Part model, mm, in its own coordinate system. A direction names the side the tool comes from. Round coordinates to 2 decimals unless told otherwise and drop trailing zeros. Write each loop counter-clockwise with the first axis right and the second up, starting at its lowest first coordinate (ties: lowest second). Pieces come first, ordered by that corner, then holes.
from build123d import *

# Parameters (mm, degrees)
SKETCH1_W          = 50.8
SKETCH1_H          = 50.8
EXTRUDE1_DEPTH     = 7.9375
SKETCH6_R          = 11.1125
CUT_EXTRUDE2_DEPTH = 8.255
SKETCH3_R          = 6.35
EXTRUDE3_DEPTH     = 6.35
CHAMFER1_SIZE      = 9.525


with BuildPart() as part:
    # Sketch1 → Extrude1 (new body, symmetric)
    with BuildSketch(Plane.XY):
        Rectangle(SKETCH1_W, SKETCH1_H)
    extrude(amount=EXTRUDE1_DEPTH, both=True)

    # Sketch6 → Cut-Extrude2 (cut)
    with BuildSketch(Plane.XY.offset(7.9375)):
        Circle(SKETCH6_R)
    extrude(amount=-CUT_EXTRUDE2_DEPTH, mode=Mode.SUBTRACT)

    # Sketch3 → Extrude3 (add)
    with BuildSketch(Plane.ZY.offset(25.4)):
        with Locations(Location((0, 0, 0), (0, 0, 90))):  # turned: the seam where the file's is
            Circle(SKETCH3_R)
    extrude3 = extrude(amount=EXTRUDE3_DEPTH)

    # Mirror2: Extrude3 across plane
    add(extrude3.mirror(Plane(origin=(0, 0, 0), x_dir=(0, 0, 1), z_dir=(1, 0, 0))))

    # Chamfer1
    chamfer1_edges = [part.edges().sort_by_distance(p)[0] for p in [
        (0, 25.4, -7.9375),
        (0, -25.4, -7.9375),
    ]]
    chamfer(chamfer1_edges, length=CHAMFER1_SIZE)


solid = part.part
Q1. Tool access for faces 4 (the flat face through (0, 0, -0.318)), 5 (the cylindrical face through (28.53, -5.04, 3.86)), 6 (the flat face through (-0.36, -20.57, -3.24)): list every direction of +Z, -Z, +X, -X, +Y, -Y with a clear straight run to the whole face (end or side of a thin tool).
Q2. Two-plate mould, pull along Y, no slides. Class faces 1 (the flat face through (0, 0, -7.938)), 2 (the cylindrical face through (10.6, 3.34, 3.87)), 3 (the cylindrical face through (-28.53, -5.04, 3.86)): released by +Y, released by -Y, zero draft, split by the parting line, or undercut.
Q3. Saw through at C-C, the plane y = 0. Write the cut outline in (x, z), and give its area (3 significant figures).
Q4. Wall check: line 1 (Y direction, x = 0, z = 5); line 2 (Z direction, x = 10, y = -2); line 3 (X direction, y = 5.5, z = -3.5). Give the ranges that are in metal, low to high.
Q5. Drop flat-ended pins along their axis: P1, Ø2, axis at y = -14, z = -5, coming from the +X side; P2, Ø4, axis at x = 10.5, z = -1.5, coming from the -Y side; P3, Ø1, axis at y = -9.5, z = 2.5, coming from the -X side; P4, Ø5, axis at y = 8, z = -3.5, coming from the +X side. Give the stop position or say it passes through.
Q6. Saw through at D-D, the plane z = -5.5. Write the cut outline in (x, y).
Q7. Saw through at A-A, the plane x = 0. Write the cut outline in (y, z) (1 decimal), and give its area (3 significant figures).
Computed:
1. face 4: +Z
1. face 5: +X
1. face 6: -Z, +X, -X, -Y
2. face 1: zero draft
2. face 2: undercut
2. face 3: split by the parting line
3. outline: (-31.75, -6.35) - (-25.4, -6.35) - (-25.4, -7.94) - (25.4, -7.94) - (25.4, -6.35) - (31.75, -6.35) - (31.75, 6.35) - (25.4, 6.35) - (25.4, 7.94) - (11.11, 7.94) - (11.11, -0.32) - (-11.11, -0.32) - (-11.11, 7.94) - (-25.4, 7.94) - (-25.4, 6.35) - (-31.75, 6.35) - close
3. area: 784 mm2
4. line 1: y = -25.4 to -11.11, 11.11 to 25.4
4. line 2: z = -7.94 to -0.32
4. line 3: x = -25.4 to 25.4
5. P1: stops at x = 25.4
5. P2: stops at y = -24.31
5. P3: stops at x = -25.4
5. P4: stops at x = 31.75
6. outline: (-31.75, -3.17) - (-25.4, -3.17) - (-25.4, -18.31) - (25.4, -18.31) - (25.4, -3.17) - (31.75, -3.17) - (31.75, 3.17) - (25.4, 3.17) - (25.4, 18.31) - (-25.4, 18.31) - (-25.4, 3.17) - (-31.75, 3.17) - close
7. outline: (-25.4, 1.6) - (-15.9, -7.9) - (15.9, -7.9) - (25.4, 1.6) - (25.4, 7.9) - (11.1, 7.9) - (11.1, -0.3) - (-11.1, -0.3) - (-11.1, 7.9) - (-25.4, 7.9) - close
7. area: 532 mm2
